from build123d import *

# Parameters (mm, degrees)
SKETCH2_R           = 9.75
SKETCH2_R_2         = 1.5
BOSS_EXTRUDE1_DEPTH = 0.5
BOSS_EXTRUDE2_START = 3.2
SKETCH3_R           = 9.75
BOSS_EXTRUDE2_DEPTH = 3.2


with BuildPart() as part:
    # Sketch2 → Boss-Extrude1 (new, symmetric)
    with BuildSketch(Plane(origin=(0, 0, 0), x_dir=(1, 0, 0), z_dir=(0, 1, 0))):
        with Locations(Location((0, 0, 0), (0, 0, 270))):
            Circle(SKETCH2_R)
        with Locations(Location((0, 0, 0), (0, 0, 270))):
            Circle(SKETCH2_R_2, mode=Mode.SUBTRACT)
    extrude(amount=BOSS_EXTRUDE1_DEPTH, both=True)

    # Sketch3 → Boss-Extrude2 (add)
    with BuildSketch(Plane(origin=(0, 0.5, 0), x_dir=(1, 0, 0), z_dir=(0, 1, 0)).offset(BOSS_EXTRUDE2_START)):
        with Locations(Location((0, 0, 0), (0, 0, 270))):
            Circle(SKETCH3_R)
        with BuildLine():
            Line((0.107421435, 2.898009771), (0.338399731, 2.678709694))
            Line((0.338399731, 2.678709694), (0.61665913, 2.83367809))
            ThreePointArc((0.61665913, 2.83367809), (0.721200673, 2.808891167), (0.824752316, 2.780248841))
            Line((0.824752316, 2.780248841), (0.993936292, 2.510396512))
            Line((0.993936292, 2.510396512), (1.301992734, 2.591295993))
            ThreePointArc((1.301992734, 2.591295993), (1.397085655, 2.541289372), (1.490260976, 2.48779465))
            Line((1.490260976, 2.48779465), (1.587020181, 2.184345885))
            Line((1.587020181, 2.184345885), (1.905517346, 2.186093238))
            ThreePointArc((1.905517346, 2.186093238), (1.985186607, 2.11400902), (2.062131058, 2.039023173))
            Line((2.062131058, 2.039023173), (2.080385755, 1.721044772))
            Line((2.080385755, 1.721044772), (2.389311295, 1.643530205))
            ThreePointArc((2.389311295, 1.643530205), (2.448550984, 1.553897705), (2.504429862, 1.46213237))
            Line((2.504429862, 1.46213237), (2.443033042, 1.149604087))
            Line((2.443033042, 1.149604087), (2.722976028, 0.997698125))
            ThreePointArc((2.722976028, 0.997698125), (2.758063897, 0.896149284), (2.789366126, 0.793370413))
            Line((2.789366126, 0.793370413), (2.652175577, 0.505929549))
            Line((2.652175577, 0.505929549), (2.885546163, 0.289177003))
            ThreePointArc((2.885546163, 0.289177003), (2.894277512, 0.182092507), (2.899036259, 0.074758075))
            Line((2.899036259, 0.074758075), (2.694672167, -0.169534403))
            Line((2.694672167, -0.169534403), (2.866806821, -0.437514174))
            ThreePointArc((2.866806821, -0.437514174), (2.848633027, -0.543405812), (2.826549281, -0.648551587))
            Line((2.826549281, -0.648551587), (2.567852594, -0.834345885))
            Line((2.567852594, -0.834345885), (2.667935462, -1.136714727))
            ThreePointArc((2.667935462, -1.136714727), (2.623998452, -1.234759946), (2.576459817, -1.331110368))
            Line((2.576459817, -1.331110368), (2.279685399, -1.446732346))
            Line((2.279685399, -1.446732346), (2.301427906, -1.764491312))
            ThreePointArc((2.301427906, -1.764491312), (2.234488404, -1.84852957), (2.164481907, -1.930030589))
            Line((2.164481907, -1.930030589), (1.848277186, -1.968215294))
            Line((1.848277186, -1.968215294), (1.790313171, -2.281398419))
            ThreePointArc((1.790313171, -2.281398419), (1.704577232, -2.346149284), (1.616501638, -2.40767989))
            Line((1.616501638, -2.40767989), (1.30073492, -2.366028036))
            Line((1.30073492, -2.366028036), (1.166706475, -2.654956874))
            ThreePointArc((1.166706475, -2.654956874), (1.067561203, -2.696351809), (0.966950626, -2.734045809))
            Line((0.966950626, -2.734045809), (0.671462695, -2.615174535))
            Line((0.671462695, -2.615174535), (0.469791321, -2.861694623))
            ThreePointArc((0.469791321, -2.861694623), (0.363466377, -2.877132634), (0.25664255, -2.888621575))
            Line((0.25664255, -2.888621575), (0, -2.7))
            Line((0, -2.7), (-0.25664255, -2.888621575))
            ThreePointArc((-0.25664255, -2.888621575), (-0.363466377, -2.877132634), (-0.469791321, -2.861694623))
            Line((-0.469791321, -2.861694623), (-0.671462695, -2.615174535))
            Line((-0.671462695, -2.615174535), (-0.966950626, -2.734045809))
            ThreePointArc((-0.966950626, -2.734045809), (-1.067561203, -2.696351809), (-1.166706475, -2.654956874))
            Line((-1.166706475, -2.654956874), (-1.30073492, -2.366028036))
            Line((-1.30073492, -2.366028036), (-1.616501638, -2.40767989))
            ThreePointArc((-1.616501638, -2.40767989), (-1.704577232, -2.346149284), (-1.790313171, -2.281398419))
            Line((-1.790313171, -2.281398419), (-1.848277186, -1.968215294))
            Line((-1.848277186, -1.968215294), (-2.164481907, -1.930030589))
            ThreePointArc((-2.164481907, -1.930030589), (-2.234488404, -1.84852957), (-2.301427906, -1.764491312))
            Line((-2.301427906, -1.764491312), (-2.279685399, -1.446732346))
            Line((-2.279685399, -1.446732346), (-2.576459817, -1.331110368))
            ThreePointArc((-2.576459817, -1.331110368), (-2.623998452, -1.234759946), (-2.667935462, -1.136714727))
            Line((-2.667935462, -1.136714727), (-2.567852594, -0.834345885))
            Line((-2.567852594, -0.834345885), (-2.826549281, -0.648551587))
            ThreePointArc((-2.826549281, -0.648551587), (-2.848633027, -0.543405812), (-2.866806821, -0.437514174))
            Line((-2.866806821, -0.437514174), (-2.694672167, -0.169534403))
            Line((-2.694672167, -0.169534403), (-2.899036259, 0.074758075))
            ThreePointArc((-2.899036259, 0.074758075), (-2.894277512, 0.182092507), (-2.885546163, 0.289177003))
            Line((-2.885546163, 0.289177003), (-2.652175577, 0.505929549))
            Line((-2.652175577, 0.505929549), (-2.789366126, 0.793370413))
            ThreePointArc((-2.789366126, 0.793370413), (-2.758063897, 0.896149284), (-2.722976028, 0.997698125))
            Line((-2.722976028, 0.997698125), (-2.443033042, 1.149604087))
            Line((-2.443033042, 1.149604087), (-2.504429862, 1.46213237))
            ThreePointArc((-2.504429862, 1.46213237), (-2.448550984, 1.553897705), (-2.389311295, 1.643530205))
            Line((-2.389311295, 1.643530205), (-2.080385755, 1.721044772))
            Line((-2.080385755, 1.721044772), (-2.062131058, 2.039023173))
            ThreePointArc((-2.062131058, 2.039023173), (-1.985186607, 2.11400902), (-1.905517346, 2.186093238))
            Line((-1.905517346, 2.186093238), (-1.587020181, 2.184345885))
            Line((-1.587020181, 2.184345885), (-1.490260976, 2.48779465))
            ThreePointArc((-1.490260976, 2.48779465), (-1.397085655, 2.541289372), (-1.301992734, 2.591295993))
            Line((-1.301992734, 2.591295993), (-0.993936292, 2.510396512))
            Line((-0.993936292, 2.510396512), (-0.824752316, 2.780248841))
            ThreePointArc((-0.824752316, 2.780248841), (-0.721200673, 2.808891167), (-0.61665913, 2.83367809))
            Line((-0.61665913, 2.83367809), (-0.338399731, 2.678709694))
            Line((-0.338399731, 2.678709694), (-0.107421435, 2.898009771))
            ThreePointArc((-0.107421435, 2.898009771), (0, 2.9), (0.107421435, 2.898009771))
        make_face(mode=Mode.SUBTRACT)
    extrude(amount=-BOSS_EXTRUDE2_DEPTH)


solid = part.part
Geometry check sheet. Reference: the model listing, model coordinates, mm. Round coordinates to 2 decimals unless told otherwise and drop trailing zeros. Order: outer loops, then holes, each group sorted by start corner. A loop starts at its lowest first (then second) coordinate and runs counter-clockwise, first axis right, second up. Notation, with made-up numbers: M 63.5,-16.5 L 78.5,-16.5 A20 cw 78.5,-3.5 Z; hole C 89,61.5 d5. An arc over 180 degrees is marked long. Answer in a Markdown table with one row per item. Add a question column.
Item 1: Sectioned sample at A-A, the plane x = -4. Enter the section's corners in (y, z).
Item 2: Draft check along X on faces 1 (the face through (1.3, 0.5, 1.2)), 2 (the face through (2.3, 3.7, 2.03)), 3 (the face through (9.667, 1.629, -1.269)). Enter one of: released by +X, released by -X, zero draft, split by the parting line, or undercut.
Item 3: Sectioned sample at B-B, the plane z = -6.5. Enter the section's corners in (x, y), plus the area to 3 significant figures.
Item 4: Depth check by flat-ended pin: pin 1 Ø4 at (x, z) = (0, 0) entering from +Y; pin 2 Ø6.5 at (x, z) = (1.5, -1) entering from +Y. Enter the tip coordinate at first touch or a pass-through.
Item 5: Material ranges on L1, parallel to X at y = -0.2, z = 0; L2, parallel to X at y = 2.75, z = -0.25; L3, parallel to Z at x = 2, y = 2.7, recorded low to high. Write a range as [from, to].
Filled in:
| question | item | result |
|---|---|---|
| 1 | outline | M -0.5,-8.89 L 3.7,-8.89 L 3.7,8.89 L -0.5,8.89 Z |
| 2 | face 1 | undercut |
| 2 | face 2 | zero draft |
| 2 | face 3 | split by the parting line |
| 3 | outline | M -7.27,-0.5 L 7.27,-0.5 L 7.27,3.7 L -7.27,3.7 Z |
| 3 | area | 61.0 mm² |
| 4 | pin 1 | stops at y = 0.5 |
| 4 | pin 2 | stops at y = 3.7 |
| 5 | L1 | x = [-9.75, -1.5], [1.5, 9.75] |
| 5 | L2 | x = [-9.75, -2.89], [2.89, 9.75] |
| 5 | L3 | z = [-9.54, -2.1], [1.95, 9.54] |
